Study the drawing (mm; zero at the part's minimum x, y, z) and answer. A direction names the side the tool comes from. Round coordinates to 2 decimals unless told otherwise and drop trailing zeros. Write each loop counter-clockwise with the first axis right and the second up, starting at its lowest first coordinate (ties: lowest second). Pieces come first, ordered by that corner, then holes.
(1) A cutting plane is placed at A-A, the plane z = 28.5. Give the vertices of the cut face in (x, y).
(2) A cutting plane is placed at D-D, the plane z = 3.5. Give the vertices of the cut face in (x, y), and give its area (3 significant figures).
(3) A cutting plane is placed at C-C, the plane x = 36. Give the vertices of the cut face in (y, z).
(4) A cutting plane is placed at B-B, the plane y = 12. Give the vertices of the cut face in (x, z), and give its area (3 significant figures).
(5) For the marked faces 1 and 2, determine the directions among +Z, -Z, +X, -X, +Y, -Y from which every point of the face is accessible in a straight line to the end or side of a thin tool.
(6) Find the intervals of material crossed by probe 1 along Y at (x, z) = (18.5, 31.5); probe 2 along X at (y, z) = (9, 21), in increasing order.
(7) Each of these flat-tipped pins is pushed along its axis until it touches: pin 1 Ø6 at (x, z) = (19, 5.5) entering from -Y; pin 2 Ø13.5 at (y, z) = (8.5, 26) entering from +X; pin 3 Ø4 at (y, z) = (12, 9.95) entering from -X. Where does it stop, or does it pass through?
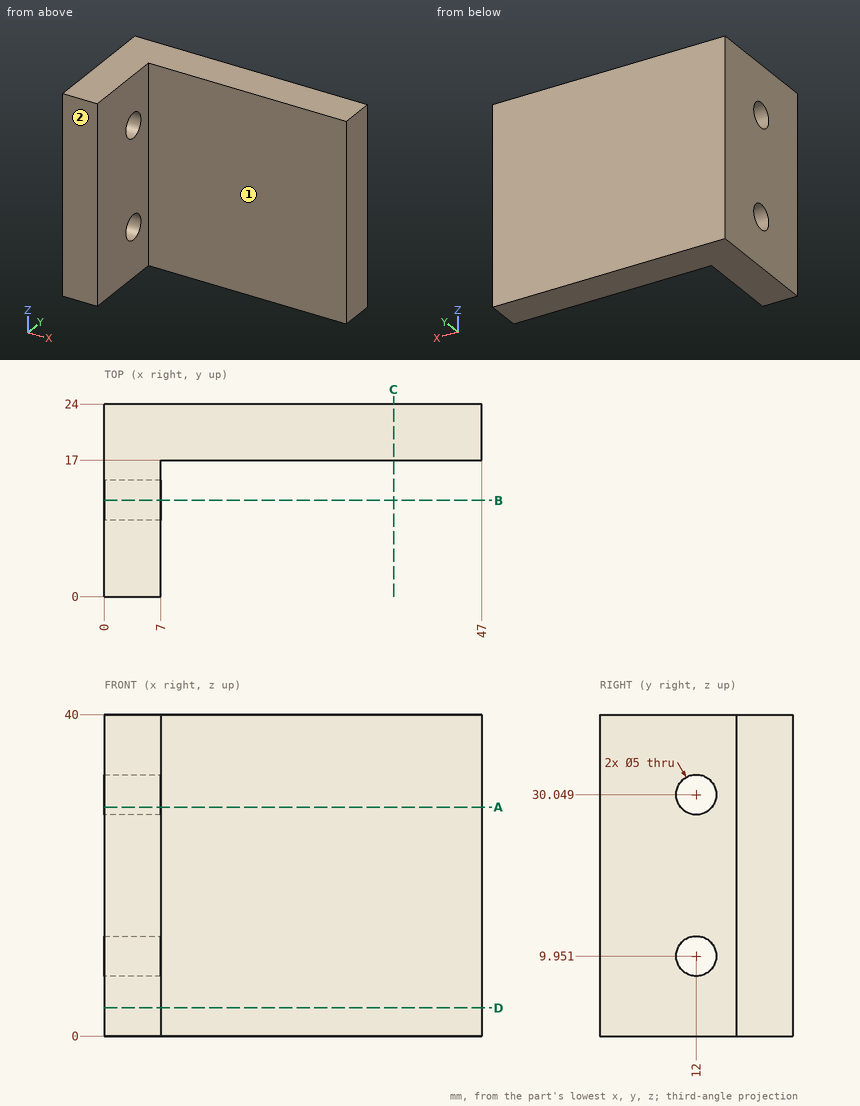
Solutions:
1. outline: (0, 0) - (7, 0) - (7, 10.04) - (0, 10.04) - close; (0, 13.96) - (7, 13.96) - (7, 17) - (47, 17) - (47, 24) - (0, 24) - close
2. outline: (0, 0) - (7, 0) - (7, 17) - (47, 17) - (47, 24) - (0, 24) - close
2. area: 448 mm2
3. outline: (17, 0) - (24, 0) - (24, 40) - (17, 40) - close
4. outline: (0, 0) - (7, 0) - (7, 7.45) - (0, 7.45) - close; (0, 12.45) - (7, 12.45) - (7, 27.55) - (0, 27.55) - close; (0, 32.55) - (7, 32.55) - (7, 40) - (0, 40) - close
4. area: 210 mm2
5. face 1: +Z, -Z, +X, -Y
5. face 2: +Z, -Z, +X, -X, -Y
6. probe 1: y = 17 to 24
6. probe 2: x = 0 to 7
7. pin 1: stops at y = 17
7. pin 2: stops at x = 7
7. pin 3: passes through
